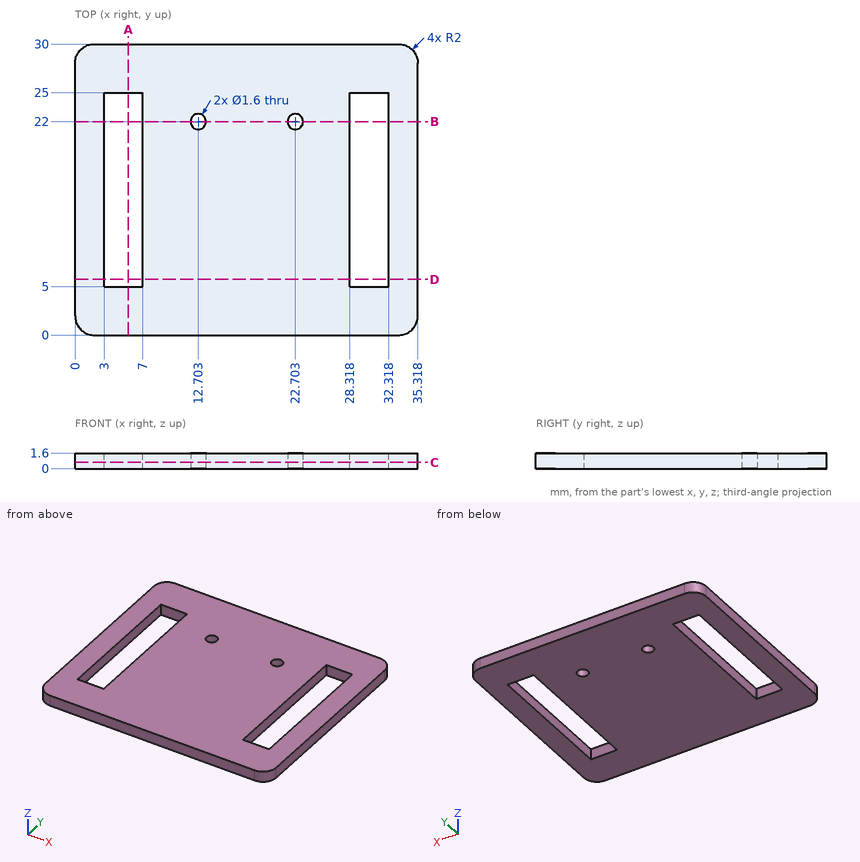
Can you work these out from the drawing? Everything is in mm from the part's minimum corner. Round coordinates to 2 decimals unless told otherwise and drop trailing zeros. Loops run counter-clockwise (first coordinate to the right, second up) from the corner with the lowest first, then second, coordinate; pieces in that order, holes last. Notation, with made-up numbers: (-7, 49) - (13, 49) arc R8 cw to (13, 64) - close; hole circle Ø3 at (-37.75, -29). An arc over 180 degrees is marked (long way). Answer in a Markdown table with one row per item. Add a question column.
(1) If we section it at B-B (y = 22): Please give me the cut outline in (x, z).
(2) I need wall thicknesses on line 1 along X through (y, z) = (21, 0.65); line 2 along Y through (x, z) = (31, 1.1); line 3 along X through (y, z) = (21.5, 0.4). Which ranges of each line are inside material? Lowest first, please.
(3) If we section it at A-A (x = 5.5): Please give me the cut outline in (y, z).
(4) If we section it at D-D (y = 5.75): Please give me the cut outline in (x, z).
(5) I'm going to push a flat-ended pin straight in: pin 1 (1.4 mm diameter, centred on x = 12.7, y = 22, fed in from +Z). Where does the tip first touch, or does it pass through?
(6) If we section it at C-C (z = 0.65): Please give me the cut outline in (x, y), plus the area to 3 significant figures.
Model answer:
| question | item | result |
|---|---|---|
| 1 | outline | (0, 0) - (3, 0) - (3, 1.6) - (0, 1.6) - close; (7, 0) - (11.9, 0) - (11.9, 1.6) - (7, 1.6) - close; (13.5, 0) - (21.9, 0) - (21.9, 1.6) - (13.5, 1.6) - close; (23.5, 0) - (28.32, 0) - (28.32, 1.6) - (23.5, 1.6) - close; (32.32, 0) - (35.32, 0) - (35.32, 1.6) - (32.32, 1.6) - close |
| 2 | line 1 | x = 0 to 3, 7 to 28.32, 32.32 to 35.32 |
| 2 | line 2 | y = 0 to 5, 25 to 30 |
| 2 | line 3 | x = 0 to 3, 7 to 12.08, 13.33 to 22.08, 23.33 to 28.32, 32.32 to 35.32 |
| 3 | outline | (0, 0) - (5, 0) - (5, 1.6) - (0, 1.6) - close; (25, 0) - (30, 0) - (30, 1.6) - (25, 1.6) - close |
| 4 | outline | (0, 0) - (3, 0) - (3, 1.6) - (0, 1.6) - close; (7, 0) - (28.32, 0) - (28.32, 1.6) - (7, 1.6) - close; (32.32, 0) - (35.32, 0) - (35.32, 1.6) - (32.32, 1.6) - close |
| 5 | pin 1 | passes through |
| 6 | outline | (0, 2) arc R2 ccw to (2, 0) - (33.32, 0) arc R2 ccw to (35.32, 2) - (35.32, 28) arc R2 ccw to (33.32, 30) - (2, 30) arc R2 ccw to (0, 28) - close; hole (3, 5) - (7, 5) - (7, 25) - (3, 25) - close; hole circle Ø1.6 at (12.7, 22); hole circle Ø1.6 at (22.7, 22); hole (28.32, 5) - (32.32, 5) - (32.32, 25) - (28.32, 25) - close |
| 6 | area | 892 mm² |
